Read the model definition and answer for the solid it produces. Units are mm, in the model's axes. Face numbers are marked on the shaded views. A direction names the side the tool comes from. Give positions to 0.01 mm unless a question says otherwise; leave off trailing zeros. Write each loop counter-clockwise with the first axis right and the second up, starting at its lowest first coordinate (ties: lowest second). Pieces come first, ordered by that corner, then holes. Notation, with made-up numbers: (75, 14.5) -> (90, 14.5) arc R25 cw to (90, 36.5) -> close; hole circle Ø8 at (65, 10.5). An arc over 180 degrees is marked (long way). Answer as CSV lines item,"result". Start each with the question number.
1. Find the intervals of material crossed by line 1 (X direction, y = -23.57, z = 142.1); line 2 (Z direction, x = -5.5, y = -28.5), in increasing order.
2. The part is cut by section A-A, the plane y = 23.57. Determine the outline of the cut face in (x, z), and give its area (3 significant figures).
3. The part is cut by section C-C, the plane z = 114.5. Determine the outline of the cut face in (x, y), and give its area (3 significant figures).
4. Given pin 1 (8 mm diameter, centred on x = 12, z = 40.5, fed in from +Y); pin 2 (6 mm diameter, centred on x = 22, z = 100, fed in from +Y); pin 3 (1.5 mm diameter, centred on x = -16, z = 25.5, fed in from -Y); pin 4 (1 mm diameter, centred on y = 17, z = 147, fed in from +X), each flat-ended and moving along its own axis, determine where each tip first touches the part or whether it passes through.
5. The part is cut by section D-D, the plane x = 12.5. Determine the outline of the cut face in (y, z).
6. A tool of negligible diameter and unlimited length cuts with its end or side. For the marked faces 1 and 2, from which of +Z, -Z, +X, -X, +Y, -Y can it reach the whole face along a straight path? Write none if from no direction.
7. The part is cut by section B-B, the plane y = 0. Determine the outline of the cut face in (x, z).
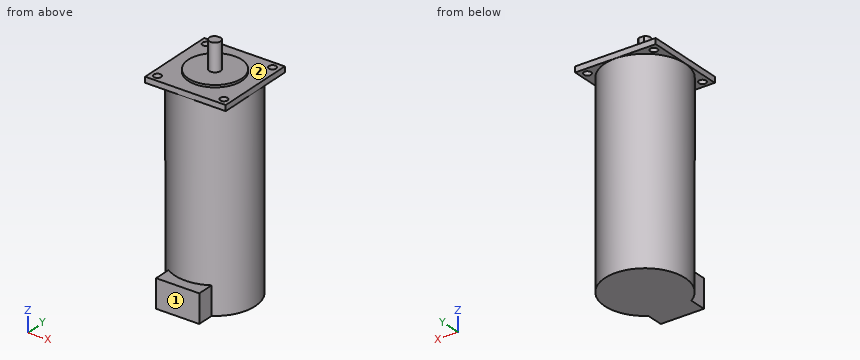
Autodesk Fusion 360 part; units mm, degrees
sketch "Sketch5" plane through (0, 0, 0) normal (0, 0, 1) x (1, 0, 0)
  circle A0 centre (0, 0) radius 28.5
  dimension "d16" = 57
extrude "Extrude5" add sketch "Sketch5" along normal blind 140
sketch "Sketch6" plane through (0, 0, 0) normal (0, 0, -1) x (1, 0, 0)
  circle A0 centre (0, 0) radius 28.5
  line L0 (0, 0) -> (0, 36)
  line L1 (0, 36) -> (-15.414, 36)
  line L2 (-15.414, 36) -> (-15.414, 23.972)
  line L3 (-15.414, 23.972) -> (0, 23.972)
  line L4 (0, 23.972) -> (0, 36)
  line L5 (-15.414, 23.972) -> (15.229, 23.972)
  line L6 (15.229, 23.972) -> (15.229, 36)
  line L7 (15.229, 36) -> (-15.414, 36)
  line L8 (-15.414, 36) -> (-15.414, 23.972)
  dimension "d19" = 36
extrude "Extrude6" add sketch "Sketch6" against normal blind 20 contours A0 L0 L1 L2 L4 L7 L8 | A0 L0 L4 L6 L7
sketch "Sketch7" plane through (0, 0, 140) normal (0, 0, 1) x (-1, 0, 0)
  circle A0 centre (0, 0) radius 28.5
  circle A1 centre (0, 0) radius 12.7
  dimension "d22" = 25.4
extrude "Extrude7" add sketch "Sketch7" along normal blind 2 contours A1
sketch "Sketch8" plane through (0, 0, 142) normal (0, 0, 1) x (-1, 0, 0)
  circle A0 centre (0, 0) radius 12.7
  circle A1 centre (0, 0) radius 4
  dimension "d25" = 8
extrude "Extrude8" add sketch "Sketch8" along normal blind 33 contours A1
sketch "Sketch9" plane through (0, 0, 175) normal (0, 0, 1) x (-1, 0, 0)
  circle A0 centre (0, 0) radius 4
  line L0 (0, 0) -> (0, 4)
  line L1 (0, 4) -> (0, -3.5)
  line L2 (0, -3.5) -> (1.9365, -3.5)
  line L3 (-1.9365, -3.5) -> (0.1996, -3.5)
  dimension "d28" = 7.5
extrude "Extrude9" cut sketch "Sketch9" against normal blind 33 contours A0 L2 L3
sketch "Sketch10" plane through (0, 0, 140) normal (0, 0, 1) x (-1, 0, 0)
  circle A0 centre (0, 0) radius 12.7
  circle A1 centre (0, 0) radius 28.5
  circle A2 centre (0, 0) radius 19.44
  line L0 (0, 0) -> (-13.7462, 13.7462)
  line L1 (0, 0) -> (19.44, 0) construction
  line L2 (-13.7462, 13.7462) -> (13.7462, -13.7462)
  line L3 (0, 0) -> (-13.7462, -13.7462)
  line L4 (0, 0) -> (13.7462, 13.7462)
  dimension "d31" = 38.88
  dimension "d32" = 135
extrude "Extrude10" cut 1 faces at (-0.3164, 6.5548, 142) along direction (0, 0, -1) blind 2
extrude "Extrude11" cut 1 faces at (0, 1, 175) along direction (0, 0, -1) blind 11
sketch "Sketch11" plane through (0, 0, 140) normal (0, 0, 1) x (-1, 0, 0)
  arc A0 (1.9365, -3.5) -> (-1.9365, -3.5) centre (0, 0) ccw
  line L0 (1.9365, -3.5) -> (-1.9365, -3.5)
  circle A1 centre (0, 0) radius 28.5
  circle A2 centre (0, 0) radius 4
  line L1 (-1.9365, -3.5) -> (1.9365, -3.5)
extrude "Extrude12" add sketch "Sketch11" along normal blind 9 contours L0 A2 L1
sketch "Sketch12" plane through (0, 0, 140) normal (0, 0, 1) x (-1, 0, 0)
  circle A0 centre (0, 0) radius 28.5
  circle A1 centre (0, 0) radius 4
  line L0 (0, 0) -> (-28.6, 0)
  line L1 (-28.6, 0) -> (-28.6, -28.6)
  line L2 (-28.6, -28.6) -> (0, -28.6)
  line L3 (0, -28.6) -> (0, 0)
  line L4 (-28.6, -28.6) -> (28.6, -28.6)
  line L5 (28.6, -28.6) -> (28.6, 28.6)
  line L6 (28.6, 28.6) -> (-28.6, 28.6)
  line L7 (-28.6, 28.6) -> (-28.6, -28.6)
  circle A2 centre (0, 0) radius 19
  dimension "d42" = 28.6
  dimension "d43" = 28.6
  dimension "d44" = 57.2
  dimension "d45" = 57.2
  dimension "d46" = 38
extrude "Extrude13" add sketch "Sketch12" along normal blind 4 contours A0 L0 L3 A2 | A0 L0 L3 L4 L5 L6 L7 | A0 L0 L3 A2 | A0 L0 L1 L2 L3 L4 L7
sketch "Sketch13" plane through (0, 0, 144) normal (0, 0, 1) x (-1, 0, 0)
  circle A0 centre (0, 0) radius 19
  line L0 (-28.6, 28.6) -> (-28.6, -28.6)
  line L1 (-28.6, -28.6) -> (28.6, -28.6)
  line L2 (28.6, -28.6) -> (28.6, 28.6)
  line L3 (28.6, 28.6) -> (-28.6, 28.6)
  line L4 (0, 0) -> (23.57, 0)
  line L5 (23.57, 0) -> (23.57, -23.57)
  line L6 (23.57, -23.57) -> (0, -23.57)
  line L7 (0, -23.57) -> (0, 0)
  line L8 (23.57, -23.57) -> (-23.57, -23.57)
  line L9 (-23.57, -23.57) -> (-23.57, 23.57)
  line L10 (-23.57, 23.57) -> (23.57, 23.57)
  line L11 (23.57, 23.57) -> (23.57, -23.57)
  circle A1 centre (23.57, -23.57) radius 2.6
  circle A2 centre (23.57, 23.57) radius 2.6
  circle A3 centre (-23.57, 23.57) radius 2.6
  circle A4 centre (-23.57, -23.57) radius 2.6
  dimension "d49" = 23.57
  dimension "d50" = 23.57
  dimension "d51" = 47.14
  dimension "d52" = 47.14
  dimension "d53" = 5.2
  dimension "d54" = 5.2
  dimension "d55" = 5.2
  dimension "d56" = 5.2
extrude "Extrude14" cut sketch "Sketch13" against normal blind 12 contours L5 L6 L8 L11 A1 | L5 L6 L8 L11 A1 | L10 L11 A2 | L10 L11 A2 | L8 L9 A4 | L8 L9 A4 | L9 L10 A3 | L9 L10 A3
extrude "Extrude15" add 1 faces at (0, -13.9646, 140) along direction (0, 0, 1) blind 6
extrude "Extrude16" cut 1 faces at (-13.9178, 1.1186, 146) along direction (0, 0, -1) blind 0.7
extrude "Extrude17" add 1 faces at (-13.9178, 1.1186, 145.3) along direction (0, 0, 1) blind 0.3
extrude "Extrude18" add 1 faces at (0, 1, 164) along direction (0, 0, 1) blind 1
extrude "Extrude19" add 1 faces at (-0.4709, 3.5807, 149) along direction (0, 0, 1) blind 1
equation "d42 = ( 57.2 / 2 ) * 1 mm"
equation "d43 = ( 57.2 / 2 ) * 1 mm"
equation "d49 = ( 47.14 / 2 ) * 1 mm"
equation "d50 = ( 47.14 / 2 ) * 1 mm"
Results found:
1,line 1,"x = -28.6 to -26.17, -20.97 to 20.97, 26.17 to 28.6"
1,line 2,"z = 0 to 20, 140 to 144"
2,outline,"(-28.6, 140) -> (-26.17, 140) -> (-26.17, 144) -> (-28.6, 144) -> close; (-20.97, 140) -> (-16.02, 140) -> (-16.02, 0) -> (16.02, 0) -> (16.02, 140) -> (20.97, 140) -> (20.97, 144) -> (-20.97, 144) -> close; (26.17, 140) -> (28.6, 140) -> (28.6, 144) -> (26.17, 144) -> close"
2,area,"4,670 mm²"
3,outline,"circle Ø57 at (0, 0)"
3,area,"2,550 mm²"
4,pin 1,"stops at y = 27.35"
4,pin 2,"stops at y = 21.24"
4,pin 3,"stops at y = -24.08"
4,pin 4,"passes through"
5,outline,"(-36, 0) -> (25.61, 0) -> (25.61, 140) -> (28.6, 140) -> (28.6, 144) -> (14.31, 144) -> (14.31, 145.6) -> (-14.31, 145.6) -> (-14.31, 144) -> (-28.6, 144) -> (-28.6, 140) -> (-25.61, 140) -> (-25.61, 20) -> (-36, 20) -> close"
6,face 1,"+Z, -Z, +X, -X, -Y"
6,face 2,"+Z"
7,outline,"(-28.6, 140) -> (-28.5, 140) -> (-28.5, 0) -> (28.5, 0) -> (28.5, 140) -> (28.6, 140) -> (28.6, 144) -> (19, 144) -> (19, 145.6) -> (4, 145.6) -> (4, 165) -> (-4, 165) -> (-4, 145.6) -> (-19, 145.6) -> (-19, 144) -> (-28.6, 144) -> close"
